Read the model definition and answer for the solid it produces. Units are mm, in the model's axes. Give positions to 0.01 mm unless a question says otherwise; leave off trailing zeros. Write each loop counter-clockwise with the first axis right and the second up, starting at its lowest first coordinate (ties: lowest second). Pieces come first, ordered by that corner, then holes. Notation, with made-up numbers: (73, 76) -> (96, 76) arc R27 ccw to (96, 115) -> close; hole circle Ø2 at (57.5, 60). An arc over 180 degrees is marked (long way). Write item = value, one per line.
from build123d import *

# Parameters (mm, degrees)
CROQUIS1_W              = 46
CROQUIS1_H              = 70
SALIENTE_EXTRUIR1_DEPTH = 1
CROQUIS2_R              = 1.5
CORTAR_EXTRUIR1_DEPTH   = 1


with BuildPart() as part:
    # Croquis1 → Saliente-Extruir1 (new body)
    with BuildSketch(Plane.XY):
        Rectangle(CROQUIS1_W, CROQUIS1_H)
    extrude(amount=SALIENTE_EXTRUIR1_DEPTH)

    # Croquis2 → Cortar-Extruir1 (cut)
    with BuildSketch(Plane.XY.offset(1)):
        with Locations((-21, -33)):
            Circle(CROQUIS2_R)
        with Locations((21, -33)):
            Circle(CROQUIS2_R)
        with Locations((-21, 33)):
            Circle(CROQUIS2_R)
        with Locations((21, 33)):
            Circle(CROQUIS2_R)
    extrude(amount=-CORTAR_EXTRUIR1_DEPTH, mode=Mode.SUBTRACT)


solid = part.part
(1) For a pull along X with two mould halves and no side action, classify faces 1 (the cylindrical face through (19.8, -33.9, 0.5)), 2 (the flat face through (0, 0, 0)) as released by +X, released by -X, zero draft, split by the parting line, or undercut.
Checks:
face_1 = undercut
face_2 = zero draft
(2) The part is cut by section B-B on x = -21. Determine the outline of the cut face in (y, z), plus the area to 3 significant figures.
Checks:
outline = (-35, 0) -> (-34.5, 0) -> (-34.5, 1) -> (-35, 1) -> close; (-31.5, 0) -> (31.5, 0) -> (31.5, 1) -> (-31.5, 1) -> close; (34.5, 0) -> (35, 0) -> (35, 1) -> (34.5, 1) -> close
area = 64.0 mm²
(3) The part is cut by section A-A on y = -33. Determine the outline of the cut face in (x, z).
Checks:
outline = (-23, 0) -> (-22.5, 0) -> (-22.5, 1) -> (-23, 1) -> close; (-19.5, 0) -> (19.5, 0) -> (19.5, 1) -> (-19.5, 1) -> close; (22.5, 0) -> (23, 0) -> (23, 1) -> (22.5, 1) -> close
(4) Consider L1, parallel to Y at x = -21, z = 0.4. Determine where the line is inside the solid, lowest interval first.
Checks:
L1 = -35 to -34.5, -31.5 to 31.5, 34.5 to 35
